Design review of the part built by this model. Coordinates are the model's own, in mm. Coordinates: 2 decimals unless noted, no trailing zeros. Write each loop counter-clockwise with the first axis right and the second up, starting at its lowest first coordinate (ties: lowest second). Pieces come first, ordered by that corner, then holes.
Q1. Take a section at C-C (x = 62). Give the boundary of the cut face in (y, z).
Q2. Insertion check: pin 1 (1.5 mm diameter, centred on x = -40, y = -101, fed in from +Z); pin 2 (4 mm diameter, centred on y = -77, z = 24.5, fed in from +X); pin 3 (2 mm diameter, centred on y = -99, z = 6, fed in from +X). Each pin has a flat end and moves straight along its axis. Give the tip position at first contact, or say it passes through.
Q3. Take a section at B-B (y = -38.5). Give the boundary of the cut face in (x, z), and give its area (3 significant figures).
Q4. For probe 1 along Y at (x, z) = (-19, 25); probe 2 along Y at (x, z) = (-58.5, 12); probe 3 along X at (y, z) = (-56, 31), list the stretches that pass through material, from the lowest coordinate up.
Q5. Take a section at A-A (z = 17). Give the boundary of the cut face in (x, y), and give its area (3 significant figures).
```python
from build123d import *

# Parameters (mm, degrees)
F1_DEPTH = 34.798
F2_SIZE  = 5.08
F3_SIZE  = 5.08


with BuildPart() as f1:
    # F0 (on Top) → F1 (new body)
    with BuildSketch(Plane.XY):
        Polygon((-110.830761, -76.057732), (69.183203, -143.250428), (104.182492, -49.48487), (-75.831473, 17.707827), align=None)
    extrude(amount=F1_DEPTH)

    # F2
    f2_edges = [f1.edges().sort_by_distance(p)[0] for p in [
        (14.17551, -15.888522, 34.798),
        (-75.831473, 17.707827, 17.399),
        (-93.331117, -29.174953, 34.798),
        (86.682848, -96.367649, 34.798),
        (-20.823779, -109.65408, 34.798),
        (104.182492, -49.48487, 17.399),
        (14.17551, -15.888522, 0),
        (-93.331117, -29.174953, 0),
        (-110.830761, -76.057732, 17.399),
        (86.682848, -96.367649, 0),
    ]]
    chamfer(f2_edges, length=F2_SIZE)

    # F3
    f3_edges = [f1.edges().sort_by_distance(p)[0] for p in [
        (-20.823779, -109.65408, 0),
    ]]
    chamfer(f3_edges, length=F3_SIZE)


solid = f1.part
```
Response:
1. outline: (-140.57, 5.08) - (-135.15, 0) - (-39.16, 0) - (-33.74, 5.08) - (-33.74, 29.72) - (-39.16, 34.8) - (-135.15, 34.8) - (-140.57, 29.72) - close
2. pin 1: stops at z = 31.87
2. pin 2: stops at x = 94.66
2. pin 3: stops at x = 86.07
3. outline: (-96.81, 5.08) - (-91.39, 0) - (60.23, 0) - (74.75, 5.08) - (74.75, 29.72) - (60.23, 34.8) - (-91.39, 34.8) - (-96.81, 29.72) - close
3. area: 5,870 mm2
4. probe 1: y = -110.33 to -3.51
4. probe 2: y = -95.59 to 11.24
4. probe 3: x = -101.98 to 100.38
5. outline: (-109.05, -71.3) - (-106.07, -77.83) - (69.18, -143.25) - (102.41, -54.24) - (99.42, -47.71) - (-71.07, 15.93) - (-77.61, 12.95) - close
5. area: 19,200 mm2
